Geometry check sheet. Reference: the model listing, model coordinates, mm. A direction names the side the tool comes from. Round coordinates to 2 decimals unless told otherwise and drop trailing zeros. Order: outer loops, then holes, each group sorted by start corner. A loop starts at its lowest first (then second) coordinate and runs counter-clockwise, first axis right, second up.
```python
from build123d import *

# Parameters (mm, degrees)
F1_R     = 5
F2_DEPTH = 20
F3_R     = 5
F4_DEPTH = 10
F7_SIZE  = 1


with BuildPart() as f2:
    # F1 (on Front) → F2 (new body)
    with BuildSketch(Plane.XZ):
        Circle(F1_R)
    extrude(amount=F2_DEPTH)

    # F3 (on face) → F4 (join)
    with BuildSketch(Plane(origin=(0, 0, 0), x_dir=(-1, 0, 0), z_dir=(0, 1, 0))):
        Polygon((4.9074772881, 8.5), (-4.9074772881, 8.5), (-9.8149545762, 0), (-4.9074772881, -8.5), (4.9074772881, -8.5), (9.8149545762, 0), align=None)
        Circle(F3_R, mode=Mode.SUBTRACT)
        Circle(F3_R)
    extrude(amount=F4_DEPTH)

    # F5 (on Right) → F6 (revolve, cut)
    with BuildSketch(Plane.YZ):
        Polygon((13.2906628903, 17.3963494964), (6.7229466513, 12.2716045007), (10, 8.0718332902), align=None)
    revolve(axis=Axis((0, 0, 0), (0, 1, 0)), mode=Mode.SUBTRACT)

    # F7
    f7_edges = [f2.edges().sort_by_distance(p)[0] for p in [
        (-5, -20, 0),
    ]]
    chamfer(f7_edges, length=F7_SIZE)


with BuildPart() as f8_1:
    # F8: copy of F2
    add(f2.part.moved(Location((25, 0, 0))))


with BuildPart() as f10_1:
    # F10: copy of F2
    add(f2.part)


with BuildPart() as f12_1:
    # F12: copy of F2
    add(f2.part.moved(Location((50, 0, 0))))


solid = f2.part
```
(1) Material ranges on line 1 (Y direction, x = 3, z = 6); line 2 (X direction, y = -8.25, z = 3), recorded low to high.
Returned:
line 1: y = 0 to 10
line 2: x = -4 to 4
(2) Depth check by flat-ended pin: P1, Ø2, axis at x = -2.5, z = 4.5, coming from the -Y side; P2, Ø3, axis at y = -12.5, z = 1.5, coming from the +X side; P3, Ø1.5, axis at x = 7, y = 2, coming from the -Z side. Enter the tip coordinate at first touch or a pass-through.
Returned:
P1: stops at y = -19.85
P2: stops at x = 5
P3: stops at z = -6.17
(3) Sectioned sample at B-B, the plane y = -15.5. Record the cut outline in (x, z), and give its area (3 significant figures).
Returned:
outline: circle Ø10 at (0, 0)
area: 78.5 mm2
(4) Set-up check for faces 1 (the cylindrical face through (-1.08, -9.37, -4.88)), 2 (the flat face through (-7.327, 4.765, -4.309)): record each of +Z, -Z, +X, -X, +Y, -Y from which the full face is reachable in a straight line by a thin tool's end or side.
Returned:
face 1: -Y
face 2: -Z, -X, +Y, -Y
(5) Sectioned sample at A-A, the plane x = 0. Record the cut outline in (y, z).
Returned:
outline: (-20, -4) - (-19, -5) - (0, -5) - (0, -8.5) - (9.67, -8.5) - (10, -8.07) - (10, 8.07) - (9.67, 8.5) - (0, 8.5) - (0, 5) - (-19, 5) - (-20, 4) - close
